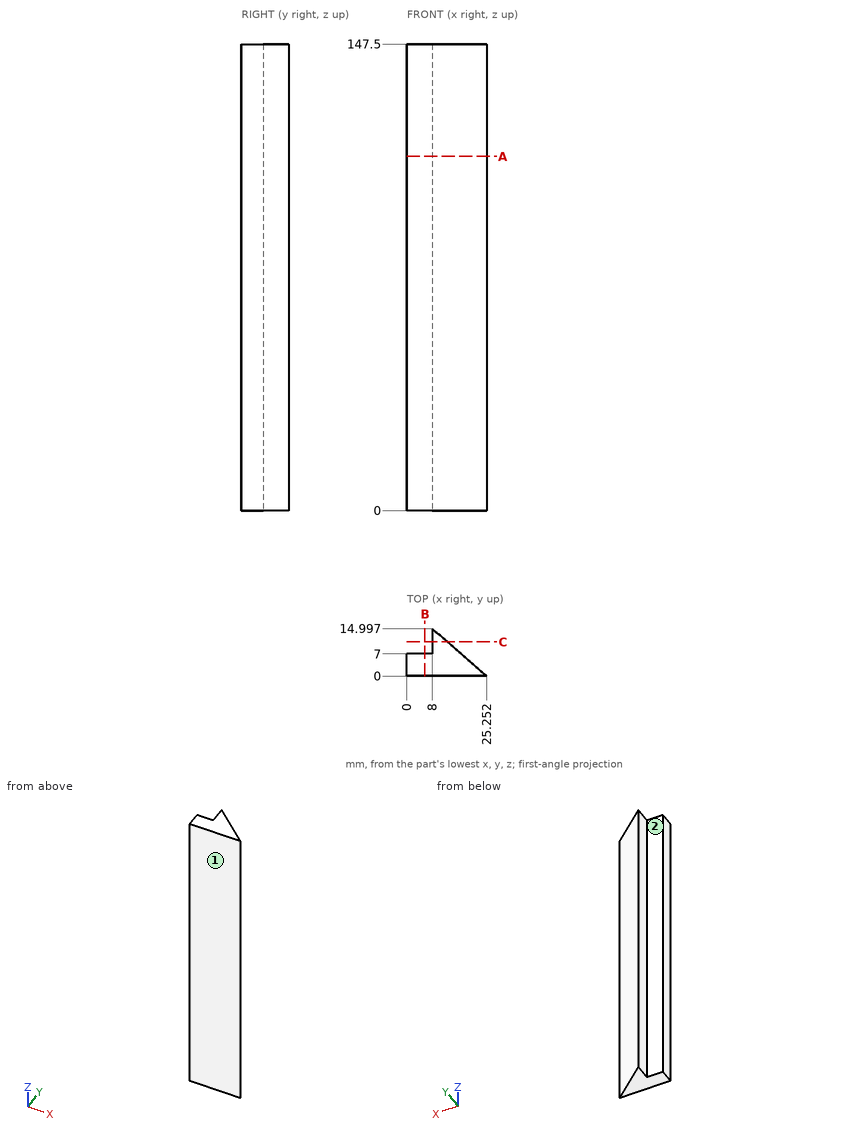
Could you check a few things on this drawing? It's one solid part, dimensions in mm from its lowest x, y, z. A direction names the side the tool comes from. Coordinates: 2 decimals unless noted, no trailing zeros. Write each loop counter-clockwise with the first axis right and the second up, starting at its lowest first coordinate (ties: lowest second). Pieces come first, ordered by that corner, then holes. Notation, with made-up numbers: (70, 31.25) - (124, 31.25) arc R14 cw to (124, 55.25) - close; hole circle Ø2 at (32.5, -20.75). An arc over 180 degrees is marked (long way). Put each result on its own line as item: value. Start each with the question number.
Q1. I'm going to push flat-ended pins straight in: P1, Ø4, axis at y = 11.5, z = 65, coming from the -X side; P2, Ø9, axis at x = 2.5, z = 48.5, coming from the +Y side; P3, Ø2, axis at y = 13, z = 86, coming from the +X side. Where does each tip first touch, or does it pass through?
Q2. I want a section at A-A on z = 112. Write out the boundary of the cut face in (x, y).
Q3. Please list where these lines run through material, in increasing order: L1, parallel to Y at x = 5.5, z = 61; L2, parallel to X at y = 9.75, z = 120 (1 decimal); L3, parallel to Y at x = 20, z = 8.5 (1 decimal).
Q4. I want a section at C-C on y = 10.75. Write out the boundary of the cut face in (x, z).
Q5. Which directions (+Z, -Z, +X, -X, +Y, -Y) give clear straight access to the entire face, cutting with the end or side of a thin tool? Please do the marked faces 1 and 2.
Q6. I want a section at B-B on x = 5.75. Write out the boundary of the cut face in (y, z).
Checks:
1. P1: x = 8
1. P2: y = 7
1. P3: x = 11.45
2. outline: (0, 0) - (25.25, 0) - (8, 15) - (8, 7) - (0, 7) - close
3. L1: 0 to 7
3. L2: 8 to 14
3. L3: 0 to 4.6
4. outline: (8, 0) - (12.89, 0) - (12.89, 147.5) - (8, 147.5) - close
5. face 1: +Z, -Z, +X, -X, -Y
5. face 2: +Z, -Z, -X, +Y
6. outline: (0, 0) - (7, 0) - (7, 147.5) - (0, 147.5) - close
